Design review of the part built by this model. Coordinates are the model's own, in mm. A direction names the side the tool comes from. Round coordinates to 2 decimals unless told otherwise and drop trailing zeros. Loops run counter-clockwise (first coordinate to the right, second up) from the corner with the lowest first, then second, coordinate; pieces in that order, holes last. Notation, with made-up numbers: (16.25, -31.5) - (61.25, -31.5) arc R22 cw to (61.25, -22.5) - close; hole circle Ø8 at (28.25, -15). An arc over 180 degrees is marked (long way). Answer as CSV lines item,"result". Start each with the question number.
(1) Mouldability with a two-part tool opening along X and no side actions: class faces 3 (the flat face through (-43.2, 0.78, -36.96)), 4 (the cylindrical face through (33.275, 0.783, -35.005)), 5 (the cylindrical face through (79.094, 0.783, 0.878)), 6 (the cylindrical face through (55.97, 0.78, 4.54)) as released by +X, released by -X, zero draft, split by the parting line, or undercut.
(2) Consider section A-A (x = 24.5). Give the boundary of the cut face in (y, z).
(3) Consider section B-B (z = -13). Give the boundary of the cut face in (x, y), and give its area (3 significant figures).
(4) For faces 1 (the cylindrical face through (-48.836, 0.783, -29.921)), 2 (the cylindrical face through (43.18, 0.78, -28.74)), list the 3-axis set-ups (+Z, -Z, +X, -X, +Y, -Y) from which the entire face can be reached by the end or side of a thin tool; tool diameter is ignored.
(5) Wall thickness on L1, parallel to Z at x = 24.5, y = 1; L2, parallel to X at y = 1.1, z = -18; L3, parallel to X at y = 0.3, z = -37.5: over which ranges is each line inside the solid? List them lowest first.
(6) Consider section C-C (y = 1.1). Give the boundary of the cut face in (x, z).
Autodesk Inventor part; units mm, degrees
ref_plane "YZ Plane" through (0, 0, 0) normal (1, 0, 0) x (0, 1, 0)
ref_plane "XZ Plane" through (0, 0, 0) normal (0, 1, 0) x (-1, 0, 0)
ref_plane "XY Plane" through (0, 0, 0) normal (0, 0, 1) x (1, 0, 0)
sketch "Sketch1" plane through (0, 0, 0) normal (0, 1, 0) x (-1, 0, 0)
  line L0 (-37.8542, -1.1176) -> (35.8058, -1.1176)
  line L1 (43.4258, -8.7376) -> (43.4258, -23.2918)
  line L2 (35.8058, -30.9118) -> (-37.8542, -30.9118)
  line L3 (-45.4742, -23.2918) -> (-45.4742, -8.7376)
  arc A0 (-37.8542, -1.1176) -> (-45.4742, -8.7376) centre (-37.8542, -8.7376) ccw
  arc A1 (-45.4742, -23.2918) -> (-37.8542, -30.9118) centre (-37.8542, -23.2918) ccw
  arc A2 (35.8058, -30.9118) -> (43.4258, -23.2918) centre (35.8058, -23.2918) ccw
  arc A3 (43.4258, -8.7376) -> (35.8058, -1.1176) centre (35.8058, -8.7376) ccw
  circle A4 centre (-72.8662, -0.3634) radius 2.3114
  circle A5 centre (-54.9057, -18.324) radius 2.3114
  circle A6 centre (-58.1742, 5.2324) radius 2.3114
  circle A7 centre (-32.7742, -37.2618) radius 2.3114
  circle A8 centre (30.7258, -37.2618) radius 2.3114
  circle A9 centre (43.4258, 5.2324) radius 2.3114
  arc A10 (49.7758, 5.2324) -> (43.4258, 11.5824) centre (43.4258, 5.2324) ccw
  arc A11 (-75.1264, 5.5707) -> (-77.3564, -4.8536) centre (-72.8662, -0.3634) ccw
  arc A12 (-58.1742, 11.5824) -> (-60.4344, 11.1665) centre (-58.1742, 5.2324) ccw
  line L4 (35.8058, -30.9118) -> (-37.8542, -30.9118)
  line L5 (-75.1264, 5.5707) -> (-60.4344, 11.1665)
  line L6 (-77.3564, -4.8536) -> (-42.3179, -39.8921)
  line L7 (-33.3376, -43.6118) -> (31.2893, -43.6118)
  line L8 (-58.1742, 11.5824) -> (43.4258, 11.5824)
  arc A13 (-42.3179, -39.8921) -> (-33.3376, -43.6118) centre (-33.3376, -30.9118) ccw
  arc A14 (35.8058, -30.9118) -> (43.4258, -23.2918) centre (35.8058, -23.2918) ccw
  line L9 (46.0561, -34.1055) -> (40.2695, -39.8921)
  arc A15 (31.2893, -43.6118) -> (40.2695, -39.8921) centre (31.2893, -30.9118) ccw
  line L10 (49.7758, 5.2324) -> (49.7758, -25.1252)
  arc A16 (46.0561, -34.1055) -> (49.7758, -25.1252) centre (37.0758, -25.1252) ccw
  point P0 (0, 0)
  point P1 (43.4258, -30.9118)
  point P2 (43.4258, -1.1176)
  point P3 (-45.4742, -30.9118)
  point P4 (43.4258, -30.9118)
  point P5 (41.194, -28.68)
  dimension "d2" = 7.62
  dimension "d21" = 12.7
extrude "Extrusion1" add sketch "Sketch1" along normal blind 1.5875
properties part number "gusset-2-3.25-full-no-front"
Determined:
1,face 3,"released by -X"
1,face 4,"undercut"
1,face 5,"released by +X"
1,face 6,"undercut"
2,outline,"(0, -43.61) - (1.59, -43.61) - (1.59, -30.91) - (0, -30.91) - close; (0, -1.12) - (1.59, -1.12) - (1.59, 11.58) - (0, 11.58) - close"
3,outline,"(-49.78, 0) - (-43.43, 0) - (-43.43, 1.59) - (-49.78, 1.59) - close; (45.47, 0) - (69.21, 0) - (69.21, 1.59) - (45.47, 1.59) - close"
3,area,"47.8 mm^2"
4,face 1,"-Z, -X, +Y, -Y"
4,face 2,"+Y, -Y"
5,L1,"z = -43.61 to -30.91, -1.12 to 11.58"
5,L2,"x = -49.78 to -43.43, 45.47 to 52.62, 57.19 to 64.21"
5,L3,"x = -42.66 to -33.02, -28.43 to 30.48, 35.07 to 44.71"
6,outline,"(-49.78, -25.13) arc R12.7 ccw to (-46.06, -34.11) - (-40.27, -39.89) arc R12.7 ccw to (-31.29, -43.61) - (33.34, -43.61) arc R12.7 ccw to (42.32, -39.89) - (77.36, -4.85) arc R6.35 ccw to (75.13, 5.57) - (60.43, 11.17) arc R6.35 ccw to (58.17, 11.58) - (-43.43, 11.58) arc R6.35 ccw to (-49.78, 5.23) - close; hole circle Ø4.62 at (-43.43, 5.23); hole (-43.43, -23.29) arc R7.62 ccw to (-35.81, -30.91) - (37.85, -30.91) arc R7.62 ccw to (45.47, -23.29) - (45.47, -8.74) arc R7.62 ccw to (37.85, -1.12) - (-35.81, -1.12) arc R7.62 ccw to (-43.43, -8.74) - close; hole circle Ø4.62 at (-30.73, -37.26); hole circle Ø4.62 at (32.77, -37.26); hole circle Ø4.62 at (54.91, -18.32); hole circle Ø4.62 at (58.17, 5.23); hole circle Ø4.62 at (72.87, -0.36)"
